```python
from build123d import *

# Parameters (mm, degrees)
SKETCH_1_W          = 250
SKETCH_1_H          = 300
EXTRUDE_1_DEPTH     = 300
SKETCH_2_W          = 230
SKETCH_2_H          = 280
CUT_EXTRUDE_1_DEPTH = 290
SKETCH_3_W          = 295
SKETCH_3_H          = 360
EXTRUDE_2_DEPTH     = 10
CUT_EXTRUDE_2_DEPTH = 15


with BuildPart() as part:
    # 草图1 → 凸台-拉伸1 (new body)
    with BuildSketch(Plane.XY):
        with Locations((125, 150)):
            Rectangle(SKETCH_1_W, SKETCH_1_H)
    extrude(amount=EXTRUDE_1_DEPTH)

    # 草图2 → 切除-拉伸1 (cut)
    with BuildSketch(Plane.XY.offset(300)):
        with Locations((125, 150)):
            Rectangle(SKETCH_2_W, SKETCH_2_H)
    extrude(amount=-CUT_EXTRUDE_1_DEPTH, mode=Mode.SUBTRACT)

    # 草图3 → 凸台-拉伸2 (add)
    with BuildSketch(Plane.XZ):
        with Locations((117.5, 150)):
            Rectangle(SKETCH_3_W, SKETCH_3_H)
    extrude(amount=EXTRUDE_2_DEPTH)

    # 草图4 → 切除-拉伸2 (cut)
    with BuildSketch(Plane.XZ.offset(10)):
        with BuildLine():
            Line((75.410884938, 284.219295629), (151.62630951, 284.219295629))
            ThreePointArc((151.62630951, 284.219295629), (165.845605139, 270), (151.62630951, 255.780704371))
            Line((151.62630951, 255.780704371), (75.410884938, 255.780704371))
            ThreePointArc((75.410884938, 255.780704371), (61.191589309, 270), (75.410884938, 284.219295629))
        make_face()
    extrude(amount=-CUT_EXTRUDE_2_DEPTH, mode=Mode.SUBTRACT)


solid = part.part
```
Could you check a few things on this model? Use its own coordinates, in mm. A direction names the side the tool comes from. Coordinates: 2 decimals unless noted, no trailing zeros. Write each loop counter-clockwise with the first axis right and the second up, starting at its lowest first coordinate (ties: lowest second). Pieces come first, ordered by that corner, then holes. Notation, with made-up numbers: (72, 68.5) -> (98, 68.5) arc R33 ccw to (98, 98.5) -> close; hole circle Ø9 at (39, 43). An arc over 180 degrees is marked (long way). Return JSON: item names as keys, results as strings.
(1) Imagine slicing it at A-A, the plane z = 76.5. Please give me the cut outline in (x, y).
Numbers:
{"outline": "(-30, -10) -> (265, -10) -> (265, 0) -> (250, 0) -> (250, 300) -> (0, 300) -> (0, 0) -> (-30, 0) -> close; hole (10, 10) -> (240, 10) -> (240, 290) -> (10, 290) -> close"}
(2) Which directions (+Z, -Z, +X, -X, +Y, -Y) give clear straight access to the entire face, cutting with the end or side of a thin tool? Please do faces 4 (the flat face through (123, 152, 0)), 5 (the flat face through (4, 151, 300)), 6 (the cylindrical face through (61.195, -2.605, 269.687)), 7 (the flat face through (123, 10, 157)).
Numbers:
{"face 4": "-Z, +X, -X, +Y", "face 5": "+Z, +X, -X, +Y", "face 6": "-Y", "face 7": "+Z"}
(3) We'd pull the mould along X, two halves only. Please class faces 1 (the flat face through (114, -3, 255.781)), 2 (the flat face through (265, -5, 147)), 3 (the flat face through (-3, 0, 151)): +X half, -X half, draft (parallel to the pull), parting line (faces both ways), or undercut.
Numbers:
{"face 1": "undercut", "face 2": "+X half", "face 3": "draft"}
(4) I need wall thicknesses on L1, parallel to Y at x = 37, z = 170; L2, parallel to X at y = 120.5, z = 134; L3, parallel to Y at x = 163, z = 269. Which ranges of each line are inside material? Lowest first, please.
Numbers:
{"L1": "y = -10 to 10, 290 to 300", "L2": "x = 0 to 10, 240 to 250", "L3": "y = 5 to 10, 290 to 300"}
(5) Imagine slicing it at D-D, the plane x = 204.5. Please give me the cut outline in (y, z), then the cut area to 3 significant figures.
Numbers:
{"outline": "(-10, -30) -> (0, -30) -> (0, 0) -> (300, 0) -> (300, 300) -> (290, 300) -> (290, 10) -> (10, 10) -> (10, 300) -> (0, 300) -> (0, 330) -> (-10, 330) -> close", "area": "12,400 mm2"}
(6) I'm going to push flat-ended pins straight in: pin 1 (8.5 mm diameter, centred on x = 127.5, z = 266.5, fed in from -Y); pin 2 (1.5 mm diameter, centred on y = 81, z = 194, fed in from -X); pin 3 (5 mm diameter, centred on y = 175.5, z = 61, fed in from +X). Where does each tip first touch, or does it pass through?
Numbers:
{"pin 1": "stops at y = 5", "pin 2": "stops at x = 0", "pin 3": "stops at x = 250"}
(7) Imagine slicing it at B-B, the plane x = 142. Please give me the cut outline in (y, z), then the cut area to 3 significant figures.
Numbers:
{"outline": "(-10, -30) -> (0, -30) -> (0, 0) -> (300, 0) -> (300, 300) -> (290, 300) -> (290, 10) -> (10, 10) -> (10, 300) -> (0, 300) -> (0, 330) -> (-10, 330) -> (-10, 284.22) -> (5, 284.22) -> (5, 255.78) -> (-10, 255.78) -> close", "area": "12,000 mm2"}
(8) Imagine slicing it at C-C, the plane z = 270. Please give me the cut outline in (x, y).
Numbers:
{"outline": "(-30, -10) -> (61.19, -10) -> (61.19, 5) -> (165.85, 5) -> (165.85, -10) -> (265, -10) -> (265, 0) -> (250, 0) -> (250, 300) -> (0, 300) -> (0, 0) -> (-30, 0) -> close; hole (10, 10) -> (240, 10) -> (240, 290) -> (10, 290) -> close"}
